Input: part model. Units: mm. Frame: model coordinates. A direction names the side the tool comes from. Round coordinates to 2 decimals unless told otherwise and drop trailing zeros. Loops run counter-clockwise (first coordinate to the right, second up) from the corner with the lowest first, then second, coordinate; pieces in that order, holes last. Notation, with made-up numbers: (78.5, -32.75) -> (93.5, -32.75) arc R29 cw to (93.5, 4.25) -> close; hole circle Ø7 at (35, 55.25). An arc over 180 degrees is marked (long way). Answer in a Markdown table with one row per item. Add a question column.
Q1. Pin query (flat end, axial travel): pin 1 (1.7 mm diameter, centred on x = -9.5, y = 9, fed in from +Z); pin 2 (2.5 mm diameter, centred on x = -45, y = 0, fed in from -Z); pin 3 (5 mm diameter, centred on y = 9.5, z = 2.5, fed in from -X); pin 4 (1.5 mm diameter, centred on y = 14, z = 7.5, fed in from -X). Return the tip coordinate at first contact, or that it passes through.
Q2. Ray query, L1, parallel to Y at x = -10, z = 3.9; L2, parallel to X at y = 17.5, z = 2.5; L3, parallel to Z at x = -41, y = -9.5. Return the intervals inside material, ascending. Write a range as from..to.
Q3. Section A-A, the plane y = 0. Output: boundary loops of the cut face in (x, z), and give its area (3 significant figures).
Q4. Section B-B, the plane z = 1.75. Give the number of separate pieces and of enclosed holes in the cut face, and give its area (3 significant figures).
Q5. Section C-C, the plane y = -19. Output: boundary loops of the cut face in (x, z), and give its area (3 significant figures).
Q6. Mould query, pull axis Y, two halves, no side actions, for faces 1 (the face through (-19.1, 24.14, 2.54)), 2 (the face through (-42.95, 0.65, 2.46)), 3 (the face through (15, 0, 2)). Classes: pulls with the +Y half, pulls with the -Y half, needs draft (parallel to the pull), parting line crosses it, or undercut.
Q7. Reachability of faces 4 (the face through (-13, 19, 5)), 5 (the face through (-14, 0, 0)), 6 (the face through (-20, -16, 2)), 7 (the face through (-11.6, 10.07, 1.48)), 8 (the face through (-10.693, 14.564, 9.248)) from +Z, -Z, +X, -X, +Y, -Y: full face, straight path, thin tool, end or side. Return the list, or none.
```python
from build123d import *

# Parameters (mm, degrees)
SKETCH_R        = 1.6
SKETCH_R_2      = 2.15
SKETCH_R_3      = 2.2
PAD_DEPTH       = 5
SKETCH001_R     = 2.9
POCKET_DEPTH    = 2
SKETCH002_R     = 5
PAD001_DEPTH    = 8
SKETCH003_R     = 2.2
POCKET001_DEPTH = 3
FILLET_R        = 0.6
FILLET001_R     = 3
FILLET002_R     = 3


with BuildPart() as part:
    # Sketch → Pad (new body)
    with BuildSketch(Plane.XY):
        Polygon((-20, 25), (15, 25), (15, -25), (-20, -25), (-20, -10), (-60, -10), (-60, 10), (-20, 10), align=None)
        with Locations((-10, 10)):
            Circle(SKETCH_R, mode=Mode.SUBTRACT)
        with Locations((10, 10)):
            Circle(SKETCH_R, mode=Mode.SUBTRACT)
        with Locations((10, -10)):
            Circle(SKETCH_R, mode=Mode.SUBTRACT)
        with Locations((-10, -10)):
            Circle(SKETCH_R, mode=Mode.SUBTRACT)
        with Locations((-20, 0)):
            Circle(SKETCH_R_2, mode=Mode.SUBTRACT)
        with Locations((-45, 0)):
            Circle(SKETCH_R_2, mode=Mode.SUBTRACT)
        with Locations((-13, 19)):
            Circle(SKETCH_R_3, mode=Mode.SUBTRACT)
        with Locations((-13, -19)):
            Circle(SKETCH_R_3, mode=Mode.SUBTRACT)
    extrude(amount=PAD_DEPTH)

    # Sketch001 → Pocket (cut)
    with BuildSketch(Plane.XY.offset(5)):
        with Locations((-10, 10)):
            Circle(SKETCH001_R)
        with Locations((10, 10)):
            Circle(SKETCH001_R)
        with Locations((10, -10)):
            Circle(SKETCH001_R)
        with Locations((-10, -10)):
            Circle(SKETCH001_R)
    extrude(amount=-POCKET_DEPTH, mode=Mode.SUBTRACT)

    # Sketch002 → Pad001 (new body)
    with BuildSketch(Plane.XY.offset(5)):
        with Locations((-13, 19)):
            Circle(SKETCH002_R)
    extrude(amount=PAD001_DEPTH)

    # Sketch003 → Pocket001 (cut)
    with BuildSketch(Plane.XY.offset(13)):
        with Locations((-13, 19)):
            Circle(SKETCH003_R)
    extrude(amount=-POCKET001_DEPTH, mode=Mode.SUBTRACT)

    # Fillet
    fillet_edges = [part.edges().sort_by_distance(p)[0] for p in [
        (-18, 19, 5),
    ]]
    fillet(fillet_edges, radius=FILLET_R)

    # Fillet001
    fillet001_edges = [part.edges().sort_by_distance(p)[0] for p in [
        (-20, -25, 2.5),
        (-20, 25, 2.5),
        (15, 25, 2.5),
        (15, -25, 2.5),
    ]]
    fillet(fillet001_edges, radius=FILLET001_R)

    # Fillet002
    fillet002_edges = [part.edges().sort_by_distance(p)[0] for p in [
        (-60, 10, 2.5),
        (-60, -10, 2.5),
    ]]
    fillet(fillet002_edges, radius=FILLET002_R)


solid = part.part
```
Answer block:
| question | item | result |
|---|---|---|
| 1 | pin 1 | z = 3 |
| 1 | pin 2 | through |
| 1 | pin 3 | x = -60 |
| 1 | pin 4 | x = -15.63 |
| 2 | L1 | -25..-12.9, -7.1..7.1, 12.9..25 |
| 2 | L2 | -20..-14.61, -11.39..15 |
| 2 | L3 | 0..5 |
| 3 | outline | (-60, 0) -> (-47.15, 0) -> (-47.15, 5) -> (-60, 5) -> close; (-42.85, 0) -> (-22.15, 0) -> (-22.15, 5) -> (-42.85, 5) -> close; (-17.85, 0) -> (15, 0) -> (15, 5) -> (-17.85, 5) -> close |
| 3 | area | 332 mm^2 |
| 4 | separate pieces | 1 |
| 4 | enclosed holes | 8 |
| 4 | area | 2,450 mm^2 |
| 5 | outline | (-20, 0) -> (-15.2, 0) -> (-15.2, 5) -> (-20, 5) -> close; (-10.8, 0) -> (15, 0) -> (15, 5) -> (-10.8, 5) -> close |
| 5 | area | 153 mm^2 |
| 6 | face 1 | pulls with the +Y half |
| 6 | face 2 | undercut |
| 6 | face 3 | needs draft |
| 7 | face 4 | -Z |
| 7 | face 5 | -Z, +X, -X, +Y, -Y |
| 7 | face 6 | +Z, -Z, -X, -Y |
| 7 | face 7 | +Z, -Z |
| 7 | face 8 | +Z |
